```python
from build123d import *

# Parameters (mm, degrees)
BOSS_EXTRUDE1_DEPTH       = 50.8
FILLET1_R                 = 50.8
SHELL1_T                  = -2.54
SKETCH2_W                 = 45.72
SKETCH2_H                 = 45.72
CUT_EXTRUDE1_DEPTH        = 50.8
F_97_0_5_DIAMETER_HOLE1_D = 12.7
F_97_0_5_DIAMETER_HOLE2_D = 12.7


with BuildPart() as part:
    # Sketch1 → Boss-Extrude1 (new body)
    with BuildSketch(Plane.XY):
        Polygon((0, 0), (0, 1143), (520.7, 1143), (520.7, 1092.2), (50.8, 1092.2), (50.8, 0), align=None)
    extrude(amount=BOSS_EXTRUDE1_DEPTH)

    # Fillet1
    fillet1_edges = [part.edges().sort_by_distance(p)[0] for p in [
        (0, 1143, 25.4),
        (50.8, 1092.2, 25.4),
    ]]
    fillet(fillet1_edges, radius=FILLET1_R)

    # Shell1
    shell1_openings = [part.faces().sort_by_distance(p)[0] for p in [
        (520.7, 1117.6, 25.4),
    ]]
    offset(amount=SHELL1_T, openings=shell1_openings, kind=Kind.INTERSECTION)

    # Sketch2 → Cut-Extrude1 (cut)
    with BuildSketch(Plane.XZ):
        with Locations((25.4, 25.4)):
            Rectangle(SKETCH2_W, SKETCH2_H)
    extrude(amount=-CUT_EXTRUDE1_DEPTH, mode=Mode.SUBTRACT)

    # #97 (0.5) Diameter Hole1 (through all)
    with Locations(Plane(origin=(476.25, 1143, 25.4), x_dir=(0, 0, 1), z_dir=(0, 1, 0))):
        with Locations((0, 0)):
            Hole(F_97_0_5_DIAMETER_HOLE1_D / 2)

    # #97 (0.5) Diameter Hole2 (through all)
    with Locations(Plane(origin=(25.4, 101.6, 50.8), x_dir=(1, 0, 0), z_dir=(0, 0, 1))):
        with Locations((0, 0), (0, 165.1)):
            Hole(F_97_0_5_DIAMETER_HOLE2_D / 2)


solid = part.part
```
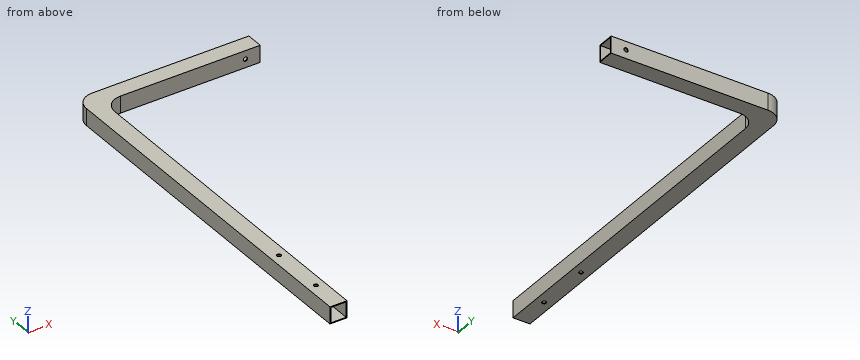
CAD build for the part. Positions are in the model's coordinates, mm. Round coordinates to 2 decimals unless told otherwise and drop trailing zeros. Write each loop counter-clockwise with the first axis right and the second up, starting at its lowest first coordinate (ties: lowest second). Pieces come first, ordered by that corner, then holes. Notation, with made-up numbers: (34, 74.25) - (48, 74.25) arc R14 cw to (48, 90.25) - close; hole circle Ø11 at (30.25, 47). An arc over 180 degrees is marked (long way). Return JSON: item names as keys, results as strings. Group by question number.
Item 1: Band-saw the part on A-A on y = 957. List the corners of the cut face in (x, z), plus the area to 3 significant figures.
Item 2: Flat gauge pins, fed straight in: pin 1 Ø11.5 at (x, y) = (25.4, 101.6) entering from +Z; pin 2 Ø12 at (y, z) = (282, 17) entering from +X; pin 3 Ø23 at (x, z) = (193, 26) entering from -Y. Where does each tip first touch, or does it go through?
Item 3: Band-saw the part on B-B on x = 347.5. List the corners of the cut face in (y, z).
Item 4: Probe probe 1 along Y at (x, z) = (292.5, 21); probe 2 along X at (y, z) = (266.7, 1.8). List the from-to ranges inside material, lowest first.
Resolved:
{
 "1": {"outline": "(0, 0) - (50.8, 0) - (50.8, 50.8) - (0, 50.8) - close; hole (2.54, 2.54) - (48.26, 2.54) - (48.26, 48.26) - (2.54, 48.26) - close", "area": "490 mm²"},
 "2": {"pin 1": "passes through", "pin 2": "stops at x = 50.8", "pin 3": "stops at y = 1092.2"},
 "3": {"outline": "(1092.2, 0) - (1143, 0) - (1143, 50.8) - (1092.2, 50.8) - close; hole (1094.74, 2.54) - (1140.46, 2.54) - (1140.46, 48.26) - (1094.74, 48.26) - close"},
 "4": {"probe 1": "y = 1092.2 to 1094.74, 1140.46 to 1143", "probe 2": "x = 0 to 19.05, 31.75 to 50.8"}
}
